Autodesk Inventor part; units mm, degrees
ref_plane "Work Plane3" through (0, 0, 19.2) normal (0, 0, -1) x (-1, 0, 0)
ref_plane "YZ Plane" through (0, 0, 0) normal (1, 0, 0) x (0, 1, 0)
ref_plane "XZ Plane" through (0, 0, 0) normal (0, 1, 0) x (-1, 0, 0)
sketch "Sketch3" plane through (0, 0, 0) normal (0, 0, 1) x (1, 0, 0)
  circle A0 centre (0, 0) radius 9.5
  dimension "d3" = 19
extrude "Extrusion2" add sketch "Sketch3" along normal blind 22.4
sketch "Sketch4" plane through (0, 0, 22.4) normal (0, 0, 1) x (1, 0, 0)
  circle A0 centre (0, 0) radius 10.95
  dimension "d6" = 21.9
extrude "Extrusion3" add sketch "Sketch4" along normal blind 2
sketch "Sketch5" plane through (0, 0, 24.4) normal (0, 0, 1) x (1, 0, 0)
  circle A0 centre (0, 0) radius 8.89
  dimension "d10" = 17.78
fillet "Fillet1" radius 1.905 1 edges at (-10.95, 0, 24.4)
ref_plane "Work Plane3" through (0, 0, 19.2) normal (0, 0, -1) x (-1, 0, 0)
sketch "Sketch6" plane through (0, 0, 19.2) normal (0, 0, -1) x (-1, 0, 0)
  line L0 (6.2278, -10.8381) -> (-6.2721, -10.8125)
  line L1 (-6.2721, -10.8125) -> (-12.5, 0.0256)
  line L2 (-12.5, 0.0256) -> (-6.2278, 10.8381)
  line L3 (-6.2278, 10.8381) -> (6.2721, 10.8125)
  line L4 (6.2721, 10.8125) -> (12.5, -0.0256)
  line L5 (12.5, -0.0256) -> (6.2278, -10.8381)
  point P0 (0, 0)
  point P1 (0, 0)
  dimension "d13" = 25
  dimension "d14" = 10.8125
extrude "Extrusion4" add sketch "Sketch6" along normal blind 3
extrude "Extrusion5" cut sketch "Sketch5" against normal blind 0.225
thread "Thread2"
properties part number "Button"
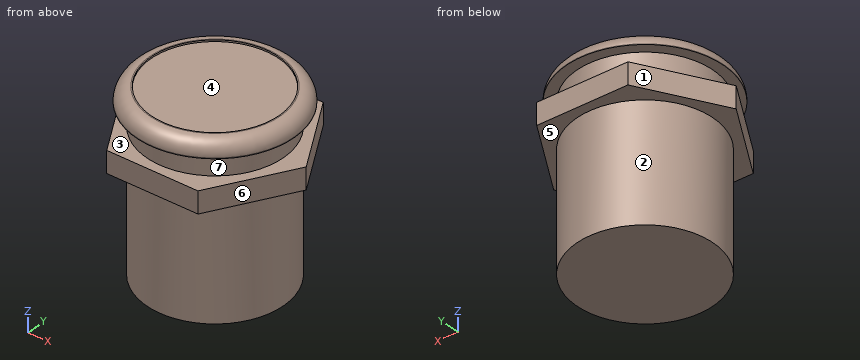
Geometry: final body of the model. Coordinates: model frame, mm. Face numbers are marked on the shaded views. A direction names the side the tool comes from. Round coordinates to 2 decimals unless told otherwise and drop trailing zeros. Order: outer loops, then holes, each group sorted by start corner. A loop starts at its lowest first (then second) coordinate and runs counter-clockwise, first axis right, second up.
Q1. Access query for the marked faces 1, 2 and 3. Directions: +Z, -Z, +X, -X, +Y, -Y. A direction counts if a zero-diameter tool reaches every point of the face in a straight line with its end or side. Return the directions, or none.
Result sheet:
face 1: -Z, -X, +Y
face 2: -Z
face 3: none
Q2. Pin query (flat end, axial travel): pin 1 (3 mm diameter, centred on x = 0.5, y = 8, fed in from +Z); pin 2 (6.5 mm diameter, centred on x = 2, y = -4, fed in from +Z) (3 decimals); pin 3 (4 mm diameter, centred on x = -4, z = 12, fed in from -Y); pin 4 (2 mm diameter, centred on x = -4, z = 20, fed in from -Y). Return the tip coordinate at first contact, or that it passes through.
Result sheet:
pin 1: stops at z = 24.4
pin 2: stops at z = 24.175
pin 3: stops at y = -9.29
pin 4: stops at y = -10.83
Q3. Section A-A, the plane x = 0. Output: boundary loops of the cut face in (y, z) (3 decimals).
Result sheet:
outline: (-10.95, 22.4) - (-9.5, 22.4) - (-9.5, 19.2) - (-10.825, 19.2) - (-10.825, 16.2) - (-9.5, 16.2) - (-9.5, 0) - (9.5, 0) - (9.5, 16.2) - (10.825, 16.2) - (10.825, 19.2) - (9.5, 19.2) - (9.5, 22.4) - (10.95, 22.4) - (10.95, 22.495) arc R1.905 ccw to (9.045, 24.4) - (8.89, 24.4) - (8.89, 24.175) - (-8.89, 24.175) - (-8.89, 24.4) - (-9.045, 24.4) arc R1.905 ccw to (-10.95, 22.495) - close
Q4. Mould query, pull axis Y, two halves, no side actions, for the marked faces 4, 5, 6 and 7. Classes: released by +Y, released by -Y, zero draft, split by the parting line, or undercut.
Result sheet:
face 4: undercut
face 5: zero draft
face 6: released by -Y
face 7: split by the parting line
Q5. Section B-B, the plane z = 5.25. Output: boundary loops of the cut face in (x, y).
Result sheet:
outline: circle Ø19 at (0, 0)
Q6. Material intervals for probe 1 along Z at (x, y) = (-2, -3) (3 decimals); probe 2 along Z at (x, y) = (9.75, 1.75); probe 3 along Z at (x, y) = (-7.25, 8.5), sorted ascending.
Result sheet:
probe 1: z = 0 to 24.175
probe 2: z = 16.2 to 19.2, 22.4 to 24.19
probe 3: z = 16.2 to 19.2
